```python
from build123d import *

# Parameters (mm, degrees)
F0_R     = 30.1625
F0_R_2   = 26.2509
F1_DEPTH = 508
F2_R     = 15.24
F4_DEPTH = 106.83089
F3_R     = 15.24
F5_DEPTH = 102.80304


with BuildPart() as f1:
    # F0 (on Top) → F1 (new body)
    with BuildSketch(Plane.XY):
        Circle(F0_R)
        Circle(F0_R_2, mode=Mode.SUBTRACT)
    extrude(amount=F1_DEPTH)

    # F2 (on Front) → F4 (cut)
    with BuildSketch(Plane.XZ):
        with Locations((0, 381)):
            Circle(F2_R)
    extrude(amount=-F4_DEPTH, mode=Mode.SUBTRACT)

    # F3 (on Front) → F5 (cut)
    with BuildSketch(Plane.XZ):
        with Locations((0, 177.8)):
            Circle(F3_R)
    extrude(amount=-F5_DEPTH, mode=Mode.SUBTRACT)


solid = f1.part
```
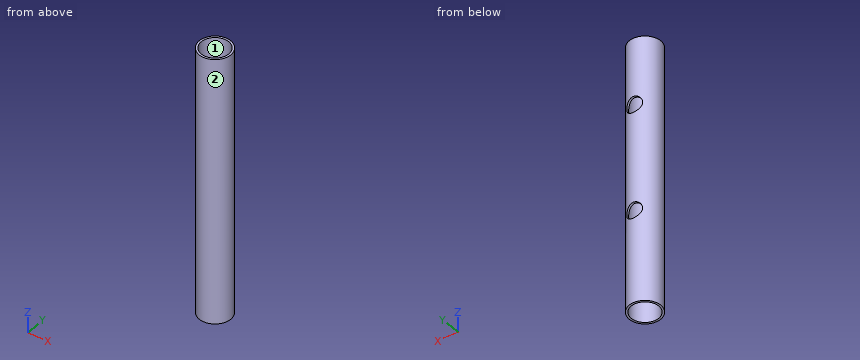
Input: part model. Units: mm. Frame: model coordinates. Face numbers are marked on the shaded views. Give positions to 0.01 mm unless a question says otherwise; leave off trailing zeros. Order: outer loops, then holes, each group sorted by start corner. A loop starts at its lowest first (then second) coordinate and runs counter-clockwise, first axis right, second up.
1. Cut plane D-D (z = 177.8). Return loops of the section in (x, y) (1 decimal), and give its area (3 significant figures).
Computed:
outline: (-15.2, 21.4) - (-15.2, 26) arc R30.2 ccw (long way) to (15.2, 26) - (15.2, 21.4) arc R26.3 cw (long way) to start
area: 567 mm2
2. Cut plane C-C (z = 265.5). Return loops of the section in (x, y) (1 decimal).
Computed:
outline: circle Ø60.3 at (0, 0); hole circle Ø52.5 at (0, 0)
3. Cut plane B-B (x = 0). Return loops of the section in (y, z), and give its area (3 significant figures).
Computed:
outline: (-30.16, 0) - (-26.25, 0) - (-26.25, 508) - (-30.16, 508) - close; (26.25, 0) - (30.16, 0) - (30.16, 162.56) - (26.25, 162.56) - close; (26.25, 193.04) - (30.16, 193.04) - (30.16, 365.76) - (26.25, 365.76) - close; (26.25, 396.24) - (30.16, 396.24) - (30.16, 508) - (26.25, 508) - close
area: 3,740 mm2
4. Cut plane A-A (y = 0). Return loops of the section in (x, z).
Computed:
outline: (-30.16, 0) - (-26.25, 0) - (-26.25, 508) - (-30.16, 508) - close; (26.25, 0) - (30.16, 0) - (30.16, 508) - (26.25, 508) - close
5. Line query: probe 1 along Z at (x, y) = (0, 27); probe 2 along Y at (x, z) = (0, 236); probe 3 along Y at (x, z) = (2, 111). Output: solid intervals per line, ascending.
Computed:
probe 1: z = 0 to 162.56, 193.04 to 365.76, 396.24 to 508
probe 2: y = -30.16 to -26.25, 26.25 to 30.16
probe 3: y = -30.1 to -26.17, 26.17 to 30.1
6. Pin query (flat end, axial travel): pin 1 Ø6 at (y, z) = (12, 396) entering from +X; pin 2 Ø2 at (y, z) = (3, 373.5) entering from -X; pin 3 Ø2 at (x, z) = (-20, 184) entering from -Y. Return the tip coordinate at first contact, or that it passes through.
Computed:
pin 1: stops at x = 28.79
pin 2: stops at x = -30.1
pin 3: stops at y = -23.43
7. Draft query along Y for the marked faces 1 and 2. Return one class per face: released by +Y, released by -Y, zero draft, split by the parting line, or undercut.
Computed:
face 1: undercut
face 2: split by the parting line
